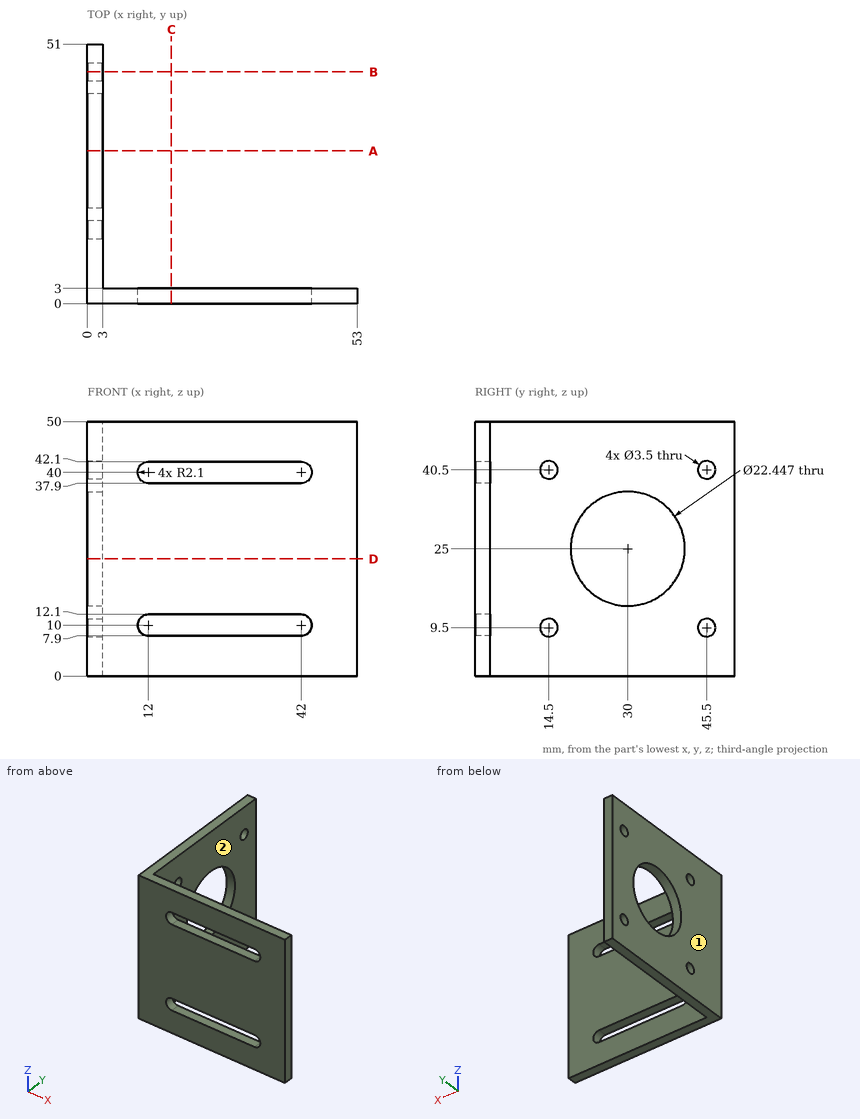
Part print with two shaded views. Sizes in mm from the minimum x, y, z corner. A direction names the side the tool comes from. Round coordinates to 2 decimals unless told otherwise and drop trailing zeros. Order: outer loops, then holes, each group sorted by start corner. A loop starts at its lowest first (then second) coordinate and runs counter-clockwise, first axis right, second up. Notation, with made-up numbers: (61, -30.75) - (116, -30.75) arc R22 cw to (116, -17.75) - close; hole circle Ø7 at (67, 89). An arc over 180 degrees is marked (long way). Return JSON: item names as keys, results as strings.
(1) Wall check: probe 1 along Z at (x, y) = (2, 45.5); probe 2 along Z at (x, y) = (37, 2.5); probe 3 along X at (y, z) = (6.5, 2). Give the ranges that are in metal, low to high. Write a range as from..to.
Answer key:
{"probe 1": "z = 0..7.75, 11.25..38.75, 42.25..50", "probe 2": "z = 0..7.9, 12.1..37.9, 42.1..50", "probe 3": "x = 0..3"}
(2) Cut at A-A (y = 30). Give the cut face in (x, z).
Answer key:
{"outline": "(0, 0) - (3, 0) - (3, 13.78) - (0, 13.78) - close; (0, 36.22) - (3, 36.22) - (3, 50) - (0, 50) - close"}
(3) Cut at C-C (x = 16.5). Give the cut face in (y, z), then the cut area to 3 significant figures.
Answer key:
{"outline": "(0, 0) - (3, 0) - (3, 7.9) - (0, 7.9) - close; (0, 12.1) - (3, 12.1) - (3, 37.9) - (0, 37.9) - close; (0, 42.1) - (3, 42.1) - (3, 50) - (0, 50) - close", "area": "125 mm^2"}
(4) Pin check, flat tips, straight feed: pin 1 Ø24 at (y, z) = (27, 31.5) entering from +X; pin 2 Ø3 at (y, z) = (45.5, 9.5) entering from -X; pin 3 Ø15 at (x, z) = (16, 30) entering from +Y. Stop position of each tip, or through.
Answer key:
{"pin 1": "stops at x = 3", "pin 2": "passes through", "pin 3": "stops at y = 3"}
(5) Cut at D-D (z = 23). Give the cut face in (x, y).
Answer key:
{"outline": "(0, 0) - (53, 0) - (53, 3) - (3, 3) - (3, 18.96) - (0, 18.96) - close; (0, 41.04) - (3, 41.04) - (3, 51) - (0, 51) - close"}
(6) Tool access for the marked faces 1 and 2: list every direction of +Z, -Z, +X, -X, +Y, -Y with a clear straight run to the whole face (end or side of a thin tool).
Answer key:
{"face 1": "+Z, -Z, -X, +Y, -Y", "face 2": "+Z, -Z, +X, +Y"}
(7) Cut at B-B (y = 45.5). Give the cut face in (x, z).
Answer key:
{"outline": "(0, 0) - (3, 0) - (3, 7.75) - (0, 7.75) - close; (0, 11.25) - (3, 11.25) - (3, 38.75) - (0, 38.75) - close; (0, 42.25) - (3, 42.25) - (3, 50) - (0, 50) - close"}
